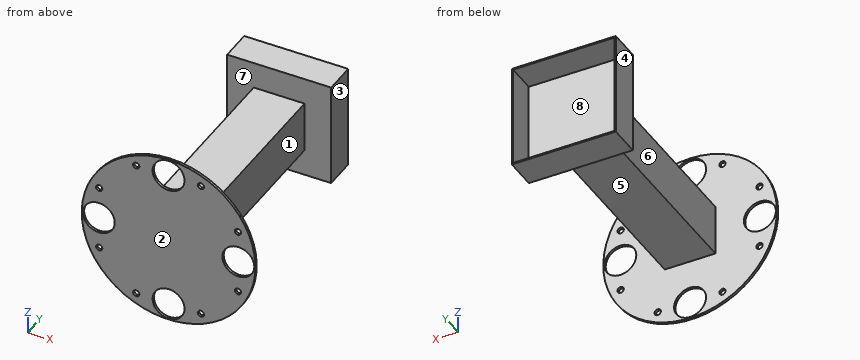
from build123d import *

# Parameters (mm, degrees)
SKETCH1_R           = 86.9315
BOSS_EXTRUDE1_DEPTH = 2.54
SKETCH2_W           = 50.8
SKETCH2_H           = 50.8
BOSS_EXTRUDE2_DEPTH = 203.2
SKETCH3_R           = 3.175
CUT_EXTRUDE1_DEPTH  = 203.2
SKETCH4_W           = 104.14
SKETCH4_H           = 104.14
BOSS_EXTRUDE3_DEPTH = 31.75
SKETCH5_W           = 101.6
SKETCH5_H           = 101.6
CUT_EXTRUDE2_DEPTH  = 29.21
SKETCH9_R           = 16.002
CUT_EXTRUDE3_DEPTH  = 266.171027611
CIRPATTERN1_COUNT   = 4


with BuildPart() as part:
    # Sketch1 → Boss-Extrude1 (new body)
    with BuildSketch(Plane(origin=(0, 0, 0), x_dir=(1, 0, 0), z_dir=(0, 1, 0))):
        with Locations(Location((0, 0, 0), (0, 0, 270))):
            Circle(SKETCH1_R)
    extrude(amount=BOSS_EXTRUDE1_DEPTH)

    # Sketch2 → Boss-Extrude2 (add)
    with BuildSketch(Plane(origin=(0, 2.54, 0), x_dir=(1, 0, 0), z_dir=(0, 1, 0))):
        Rectangle(SKETCH2_W, SKETCH2_H)
    extrude(amount=BOSS_EXTRUDE2_DEPTH)

    # Sketch3 → Cut-Extrude1 (cut)
    with BuildSketch(Plane(origin=(0, 2.54, 0), x_dir=(1, 0, 0), z_dir=(0, 1, 0))):
        with Locations(Location((-32.385, 69.50075, 0), (0, 0, 270))):
            Circle(SKETCH3_R)
        with Locations(Location((32.385, 69.50075, 0), (0, 0, 270))):
            Circle(SKETCH3_R)
        with Locations(Location((69.50075, 32.385, 0), (0, 0, 270))):
            Circle(SKETCH3_R)
        with Locations(Location((69.50075, -32.385, 0), (0, 0, 270))):
            Circle(SKETCH3_R)
        with Locations(Location((32.385, -69.50075, 0), (0, 0, 270))):
            Circle(SKETCH3_R)
        with Locations(Location((-32.385, -69.50075, 0), (0, 0, 270))):
            Circle(SKETCH3_R)
        with Locations(Location((-69.50075, -32.385, 0), (0, 0, 270))):
            Circle(SKETCH3_R)
        with Locations(Location((-69.50075, 32.385, 0), (0, 0, 270))):
            Circle(SKETCH3_R)
    extrude(amount=-CUT_EXTRUDE1_DEPTH, mode=Mode.SUBTRACT)

    # Sketch4 → Boss-Extrude3 (add)
    with BuildSketch(Plane(origin=(0, 205.74, 0), x_dir=(1, 0, 0), z_dir=(0, 1, 0))):
        Rectangle(SKETCH4_W, SKETCH4_H)
    extrude(amount=BOSS_EXTRUDE3_DEPTH)

    # Sketch5 → Cut-Extrude2 (cut)
    with BuildSketch(Plane(origin=(0, 237.49, 0), x_dir=(1, 0, 0), z_dir=(0, 1, 0))):
        Rectangle(SKETCH5_W, SKETCH5_H)
    extrude(amount=-CUT_EXTRUDE2_DEPTH, mode=Mode.SUBTRACT)

    # Sketch9 → Cut-Extrude3 (cut, through all)
    with BuildSketch(Plane(origin=(0, 2.54, 0), x_dir=(1, 0, 0), z_dir=(0, 1, 0))):
        with Locations(Location((69.85, 0, 0), (0, 0, 270))):
            Circle(SKETCH9_R)
    cut_extrude3 = extrude(amount=-CUT_EXTRUDE3_DEPTH, mode=Mode.SUBTRACT)

    # CirPattern1: Cut-Extrude3 ×4 about axis
    cirpattern1_axis = Axis((0, 0, 0), (0, 1, 0))
    for i in range(1, CIRPATTERN1_COUNT):
        add(cut_extrude3.rotate(cirpattern1_axis, i * 360 / CIRPATTERN1_COUNT), mode=Mode.SUBTRACT)


solid = part.part
Part model, mm, in its own coordinate system. Face numbers are marked on the shaded views. A direction names the side the tool comes from. Round coordinates to 2 decimals unless told otherwise and drop trailing zeros. Order: outer loops, then holes, each group sorted by start corner. A loop starts at its lowest first (then second) coordinate and runs counter-clockwise, first axis right, second up. Notation, with made-up numbers: (31, 11) -> (70, 11) arc R25 ccw to (70, 38) -> close; hole circle Ø9 at (70, 26). An arc over 180 degrees is marked (long way). Put each result on its own line as item: value.
Q1. Band-saw the part on C-C (z = 40.5). Give the cut face in (x, y), and give its area (3 significant figures).
From the geometry:
outline: (-76.92, 0) -> (76.92, 0) -> (76.92, 2.54) -> (-76.92, 2.54) -> close; (-52.07, 205.74) -> (52.07, 205.74) -> (52.07, 237.49) -> (50.8, 237.49) -> (50.8, 208.28) -> (-50.8, 208.28) -> (-50.8, 237.49) -> (-52.07, 237.49) -> close
area: 729 mm2
Q2. Tool access for the marked faces 4, 5, 6, 7 and 8: list every direction of +Z, -Z, +X, -X, +Y, -Y with a clear straight run to the whole face (end or side of a thin tool).
From the geometry:
face 4: +Z, -Z, -X, +Y
face 5: -Z, +X, -X
face 6: +Z, -Z, -X
face 7: none
face 8: +Y
Q3. Band-saw the part on D-D (x = -48). Give the cut face in (y, z).
From the geometry:
outline: (0, -72.48) -> (2.54, -72.48) -> (2.54, 72.48) -> (0, 72.48) -> close; (205.74, -52.07) -> (237.49, -52.07) -> (237.49, -50.8) -> (208.28, -50.8) -> (208.28, 50.8) -> (237.49, 50.8) -> (237.49, 52.07) -> (205.74, 52.07) -> close
Q4. Pin check, flat tips, straight feed: pin 1 Ø14.5 at (y, z) = (221, -17) entering from -X; pin 2 Ø8 at (x, z) = (39.5, 24) entering from +Y; pin 3 Ø5 at (x, z) = (21, 11) entering from -Y; pin 4 Ø5 at (x, z) = (56, 31.5) entering from +Y. Stop position of each tip, or through.
From the geometry:
pin 1: stops at x = -52.07
pin 2: stops at y = 208.28
pin 3: stops at y = 0
pin 4: stops at y = 2.54
Q5. Band-saw the part on B-B (z = 0). Give the cut face in (x, y).
From the geometry:
outline: (-86.93, 0) -> (-85.85, 0) -> (-85.85, 2.54) -> (-86.93, 2.54) -> close; (-53.85, 0) -> (53.85, 0) -> (53.85, 2.54) -> (25.4, 2.54) -> (25.4, 205.74) -> (52.07, 205.74) -> (52.07, 237.49) -> (50.8, 237.49) -> (50.8, 208.28) -> (-50.8, 208.28) -> (-50.8, 237.49) -> (-52.07, 237.49) -> (-52.07, 205.74) -> (-25.4, 205.74) -> (-25.4, 2.54) -> (-53.85, 2.54) -> close; (85.85, 0) -> (86.93, 0) -> (86.93, 2.54) -> (85.85, 2.54) -> close
Q6. Wall check: line 1 (X direction, y = 1, z = 0); line 2 (Z direction, x = 20.5, y = 225.5); line 3 (Y direction, x = 34.5, z = -27). Give the ranges that are in metal, low to high. Write a range as [from, to].
From the geometry:
line 1: x = [-86.93, -85.85], [-53.85, 53.85], [85.85, 86.93]
line 2: z = [-52.07, -50.8], [50.8, 52.07]
line 3: y = [0, 2.54], [205.74, 208.28]
Q7. Pull direction Y, two halves, no side cores. Call the marked faces 1, 2 and 3: pulls with the +Y half, pulls with the -Y half, needs draft (parallel to the pull), parting line crosses it, or undercut.
From the geometry:
face 1: undercut
face 2: pulls with the -Y half
face 3: needs draft
Q8. Band-saw the part on A-A (x = 0). Give the cut face in (y, z).
From the geometry:
outline: (0, -86.93) -> (2.54, -86.93) -> (2.54, -85.85) -> (0, -85.85) -> close; (0, -53.85) -> (2.54, -53.85) -> (2.54, -25.4) -> (205.74, -25.4) -> (205.74, -52.07) -> (237.49, -52.07) -> (237.49, -50.8) -> (208.28, -50.8) -> (208.28, 50.8) -> (237.49, 50.8) -> (237.49, 52.07) -> (205.74, 52.07) -> (205.74, 25.4) -> (2.54, 25.4) -> (2.54, 53.85) -> (0, 53.85) -> close; (0, 85.85) -> (2.54, 85.85) -> (2.54, 86.93) -> (0, 86.93) -> close
